For this review, take the finished solid that the model builds, in its own axes (mm). Give positions to 0.01 mm unless a question says otherwise; leave off trailing zeros. Loops run counter-clockwise (first coordinate to the right, second up) from the corner with the lowest first, then second, coordinate; pieces in that order, holes last.
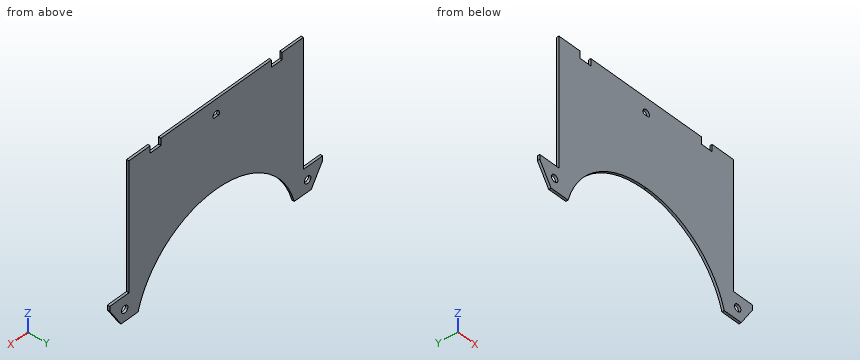
```python
from build123d import *

# Parameters (mm, degrees)
BASE_R                   = 1.5
RESSALTO_EXTRUS_O1_DEPTH = 1


with BuildPart() as part:
    # Base → Ressalto-extrusão1 (new body)
    with BuildSketch(Plane(origin=(0, 0, 0), x_dir=(1, 0, 0), z_dir=(0, 1, 0))):
        with BuildLine():
            Line((0, 56.140303816), (5.299192642, 64.620784778))
            Line((5.299192642, 64.620784778), (13.299192642, 64.620784778))
            ThreePointArc((13.299192642, 64.620784778), (27.008925086, 44.649768212), (50, 37.020302921))
            ThreePointArc((50, 37.020302921), (72.991074914, 44.649768212), (86.700807358, 64.620784778))
            Line((86.700807358, 64.620784778), (94.700807358, 64.620784778))
            Line((94.700807358, 64.620784778), (100, 56.140303816))
            Line((100, 56.140303816), (100, 54.140303816))
            Line((100, 54.140303816), (91, 54.140303816))
            Line((91, 54.140303816), (91, 0.140303816))
            Line((91, 0.140303816), (81, 0.140303816))
            Line((81, 0.140303816), (81, 3.140303816))
            Line((81, 3.140303816), (76, 3.140303816))
            Line((76, 3.140303816), (76, 0.140303816))
            Line((76, 0.140303816), (24, 0.140303816))
            Line((24, 0.140303816), (24, 3.140303816))
            Line((24, 3.140303816), (19, 3.140303816))
            Line((19, 3.140303816), (19, 0.140303816))
            Line((19, 0.140303816), (9, 0.140303816))
            Line((9, 0.140303816), (9, 54.140303816))
            Line((9, 54.140303816), (0, 54.140303816))
            Line((0, 54.140303816), (0, 56.140303816))
        make_face()
        with Locations((7, 59.640303816)):
            Circle(BASE_R, mode=Mode.SUBTRACT)
        with Locations((93, 59.640303816)):
            Circle(BASE_R, mode=Mode.SUBTRACT)
        with BuildLine():
            Line((48.781650707, 7.375), (51.218349293, 7.375))
            ThreePointArc((51.218349293, 7.375), (50, 5), (48.781650707, 7.375))
        make_face(mode=Mode.SUBTRACT)
    extrude(amount=RESSALTO_EXTRUS_O1_DEPTH)


solid = part.part
```
Item 1: Take a section at A-A on x = 93. Give the boundary of the cut face in (y, z).
Answer:
outline: (0, -64.62) - (1, -64.62) - (1, -61.14) - (0, -61.14) - close; (0, -58.14) - (1, -58.14) - (1, -54.14) - (0, -54.14) - close
Item 2: For L1, parallel to Z at x = 7, y = 0.2; L2, parallel to Z at x = 50, y = 0.4 (3 decimals); L3, parallel to X at y = 0.6, z = -6.5, list the stretches that pass through material, from the lowest coordinate up.
Answer:
L1: z = -64.62 to -61.14, -58.14 to -54.14
L2: z = -37.02 to -7.375, -5 to -0.14
L3: x = 9 to 48.5, 51.5 to 91
Item 3: Clearance check with flat-ended pins moving along their axes: pin 1 Ø0.5 at (y, z) = (0.5, -1) entering from -X; pin 2 Ø0.5 at (y, z) = (0.5, -2) entering from +X; pin 3 Ø2.5 at (x, z) = (93, -59.64) entering from -Y; pin 4 Ø0.5 at (x, y) = (95.5, 0.5) entering from +Z. State where each tip first meets the part, or that it passes through.
Answer:
pin 1: stops at x = 9
pin 2: stops at x = 91
pin 3: passes through
pin 4: stops at z = -54.14
Item 4: Take a section at D-D on z = -21. Give the boundary of the cut face in (x, y), and give its area (3 significant figures).
Answer:
outline: (9, 0) - (91, 0) - (91, 1) - (9, 1) - close
area: 82.0 mm2
Item 5: Take a section at C-C on y = 0.2. Give the boundary of the cut face in (x, z) (3 decimals).
Answer:
outline: (0, -56.14) - (5.299, -64.621) - (13.299, -64.621) arc R38 cw to (50, -37.02) arc R38 cw to (86.701, -64.621) - (94.701, -64.621) - (100, -56.14) - (100, -54.14) - (91, -54.14) - (91, -0.14) - (81, -0.14) - (81, -3.14) - (76, -3.14) - (76, -0.14) - (24, -0.14) - (24, -3.14) - (19, -3.14) - (19, -0.14) - (9, -0.14) - (9, -54.14) - (0, -54.14) - close; hole circle Ø3 at (7, -59.64); hole (48.782, -7.375) - (51.218, -7.375) arc R1.5 ccw (long way) to start; hole circle Ø3 at (93, -59.64)
Item 6: Take a section at B-B on z = -49.5. Give the boundary of the cut face in (x, y).
Answer:
outline: (9, 0) - (21.69, 0) - (21.69, 1) - (9, 1) - close; (78.31, 0) - (91, 0) - (91, 1) - (78.31, 1) - close
